For this review, take the finished solid that the model builds, in its own axes (mm). Give positions to 0.01 mm unless a question says otherwise; leave off trailing zeros. Order: outer loops, then holes, each group sorted by start corner. A loop starts at its lowest first (then second) coordinate and runs counter-clockwise, first axis right, second up. Notation, with made-up numbers: (62.5, -34) -> (121.5, -34) arc R26 cw to (121.5, -8) -> close; hole circle Ø9 at (18, 17.25). An arc over 180 degrees is marked (long way). One line per item, written item: value. Start each with the question number.
from build123d import *

# Parameters (mm, degrees)
SKETCH_1_R          = 1.5
EXTRUDE_2_DEPTH     = 3
CUT_EXTRUDE_1_DEPTH = 10
SKETCH_4_R          = 5
CUT_EXTRUDE_2_DEPTH = 10
SKETCH_5_R          = 1.5
CUT_EXTRUDE_3_DEPTH = 10
SKETCH_6_R          = 1.5
CUT_EXTRUDE_4_DEPTH = 10


with BuildPart() as part:
    # 草图1 → 凸台-拉伸2 (new body)
    with BuildSketch(Plane(origin=(0, 0, 0), x_dir=(1, 0, 0), z_dir=(0, 1, 0))):
        with BuildLine():
            Line((-60, 70), (60, 70))
            ThreePointArc((60, 70), (130, 0), (60, -70))
            Line((60, -70), (-60, -70))
            ThreePointArc((-60, -70), (-130, 0), (-60, 70))
        make_face()
        with Locations((-122, 0)):
            Circle(SKETCH_1_R, mode=Mode.SUBTRACT)
        with Locations((122, 0)):
            Circle(SKETCH_1_R, mode=Mode.SUBTRACT)
        with Locations((-30, 60)):
            Circle(SKETCH_1_R, mode=Mode.SUBTRACT)
        with Locations((30, 60)):
            Circle(SKETCH_1_R, mode=Mode.SUBTRACT)
        with Locations((30, -60)):
            Circle(SKETCH_1_R, mode=Mode.SUBTRACT)
        with Locations((-30, -60)):
            Circle(SKETCH_1_R, mode=Mode.SUBTRACT)
    extrude(amount=EXTRUDE_2_DEPTH)

    # 草图3 → 切除-拉伸1 (cut)
    with BuildSketch(Plane(origin=(0, 3, 0), x_dir=(1, 0, 0), z_dir=(0, 1, 0))):
        with BuildLine():
            Line((-60, -70), (60, -70))
            ThreePointArc((60, -70), (130, 0), (60, 70))
            Line((60, 70), (-60, 70))
            ThreePointArc((-60, 70), (-130, 0), (-60, -70))
        make_face()
        with BuildLine():
            Line((-60, -55), (60, -55))
            ThreePointArc((60, -55), (115, 0), (60, 55))
            Line((60, 55), (-60, 55))
            ThreePointArc((-60, 55), (-115, 0), (-60, -55))
        make_face(mode=Mode.SUBTRACT)
    extrude(amount=-CUT_EXTRUDE_1_DEPTH, mode=Mode.SUBTRACT)

    # 草图4 → 切除-拉伸2 (cut)
    with BuildSketch(Plane(origin=(0, 3, 0), x_dir=(1, 0, 0), z_dir=(0, 1, 0))):
        with Locations((-60, 35)):
            Circle(SKETCH_4_R)
        with Locations((-60, -35)):
            Circle(SKETCH_4_R)
        with Locations((-80.57248383, -28.315594803)):
            Circle(SKETCH_4_R)
        with Locations((-93.28697807, -10.815594803)):
            Circle(SKETCH_4_R)
        with Locations((-93.28697807, 10.815594803)):
            Circle(SKETCH_4_R)
        with Locations((-80.57248383, 28.315594803)):
            Circle(SKETCH_4_R)
        with Locations((-40, 35)):
            Circle(SKETCH_4_R)
        with Locations((-20, 35)):
            Circle(SKETCH_4_R)
        with Locations((0, 35)):
            Circle(SKETCH_4_R)
        with Locations((20, 35)):
            Circle(SKETCH_4_R)
        with Locations((40, 35)):
            Circle(SKETCH_4_R)
        with Locations((60, 35)):
            Circle(SKETCH_4_R)
        with Locations((60, -35)):
            Circle(SKETCH_4_R)
        with Locations((40, -35)):
            Circle(SKETCH_4_R)
        with Locations((20, -35)):
            Circle(SKETCH_4_R)
        with Locations((0, -35)):
            Circle(SKETCH_4_R)
        with Locations((-20, -35)):
            Circle(SKETCH_4_R)
        with Locations((-40, -35)):
            Circle(SKETCH_4_R)
        with Locations((80.57248383, 28.315594803)):
            Circle(SKETCH_4_R)
        with Locations((93.28697807, 10.815594803)):
            Circle(SKETCH_4_R)
        with Locations((93.28697807, -10.815594803)):
            Circle(SKETCH_4_R)
        with Locations((80.57248383, -28.315594803)):
            Circle(SKETCH_4_R)
    extrude(amount=-CUT_EXTRUDE_2_DEPTH, mode=Mode.SUBTRACT)

    # 草图5 → 切除-拉伸3 (cut)
    with BuildSketch(Plane(origin=(0, 3, 0), x_dir=(1, 0, 0), z_dir=(0, 1, 0))):
        with Locations((60, 51)):
            Circle(SKETCH_5_R)
        with Locations((104.167295593, 25.5)):
            Circle(SKETCH_5_R)
        with Locations((104.167295593, -25.5)):
            Circle(SKETCH_5_R)
        with Locations((60, -51)):
            Circle(SKETCH_5_R)
        with Locations((0, -51)):
            Circle(SKETCH_5_R)
        with Locations((-60, -51)):
            Circle(SKETCH_5_R)
        with Locations((-104.167295593, -25.5)):
            Circle(SKETCH_5_R)
        with Locations((-104.167295593, 25.5)):
            Circle(SKETCH_5_R)
        with Locations((-60, 51)):
            Circle(SKETCH_5_R)
        with Locations((0, 51)):
            Circle(SKETCH_5_R)
    extrude(amount=-CUT_EXTRUDE_3_DEPTH, mode=Mode.SUBTRACT)

    # 草图6 → 切除-拉伸4 (cut)
    with BuildSketch(Plane(origin=(0, 3, 0), x_dir=(1, 0, 0), z_dir=(0, 1, 0))):
        with Locations((-10, -44)):
            Circle(SKETCH_6_R)
        with Locations((-10, 44)):
            Circle(SKETCH_6_R)
        with Locations((12, -44)):
            Circle(SKETCH_6_R)
        with Locations((12, 44)):
            Circle(SKETCH_6_R)
    extrude(amount=-CUT_EXTRUDE_4_DEPTH, mode=Mode.SUBTRACT)


solid = part.part
Q1. For line 1 along Z through (x, y) = (12, 0.35); line 2 along Z through (x, y) = (57, 2.15); line 3 along X through (y, z) = (0.75, -25.5), list the stretches that pass through material, from the lowest coordinate up.
Q2. Take a section at B-B (z = -8.5). State the section outline as (x, y) points, and give its area (3 significant figures).
Q3. Take a section at A-A (x = -40). State the section outline as (y, z) points.
Q4. For pin 1 Ø8 at (x, z) = (20, -35) entering from -Y, flat-tipped, find the tip position at first contact; note if it passes through.
Q5. Mouldability with a two-part tool opening along Z and no side actions: class faces 1 (the flat face through (2, 3, -1)), 2 (the cylindrical face through (114.987, 1.521, 1.209)), 3 (the cylindrical face through (56, 2, -38)) as pulls with the +Z half, pulls with the -Z half, needs draft (parallel to the pull), parting line crosses it, or undercut.
Q6. Take a section at D-D (x = -70). State the section outline as (y, z) points, and give its area (4 significant figures).
Q7. Take a section at C-C (y = 1.3). State how many separate pieces and enclosed holes the cut face has, and give its area (3 significant figures).
Answers below:
1. line 1: z = -55 to -45.5, -42.5 to 42.5, 45.5 to 55
1. line 2: z = -55 to -39, -31 to 31, 39 to 55
1. line 3: x = -108.73 to -105.67, -102.67 to -84.7, -76.44 to 76.44, 84.7 to 102.67, 105.67 to 108.73
2. outline: (-114.34, 0) -> (-97.72, 0) -> (-97.72, 3) -> (-114.34, 3) -> close; (-88.86, 0) -> (88.86, 0) -> (88.86, 3) -> (-88.86, 3) -> close; (97.72, 0) -> (114.34, 0) -> (114.34, 3) -> (97.72, 3) -> close
2. area: 633 mm²
3. outline: (0, -55) -> (3, -55) -> (3, -40) -> (0, -40) -> close; (0, -30) -> (3, -30) -> (3, 30) -> (0, 30) -> close; (0, 40) -> (3, 40) -> (3, 55) -> (0, 55) -> close
4. pin 1: passes through
5. face 1: needs draft
5. face 2: parting line crosses it
5. face 3: undercut
6. outline: (0, -54.08) -> (3, -54.08) -> (3, 54.08) -> (0, 54.08) -> close
6. area: 324.5 mm²
7. separate pieces: 1
7. enclosed holes: 36
7. area: 20,900 mm²
